Check sheet for the modelled part. Datum: model origin and axes. Units: mm. A direction names the side the tool comes from. Give positions to 0.01 mm unless a question says otherwise; leave off trailing zeros. Order: outer loops, then holes, each group sorted by start corner. A loop starts at its lowest first (then second) coordinate and runs counter-clockwise, first axis right, second up.
from build123d import *
from build123d import SkipClean  # not in build123d's __all__

# Parameters (mm, degrees)
F0_R     = 14.2875
F1_DEPTH = 3.175
F3_DEPTH = 15.875


with BuildPart() as f1:
    # F0 (on Front) → F1 (new body)
    with BuildSketch(Plane.XZ):
        with BuildLine():
            Line((-78.184375, -32.278895576), (-12.7, -49.1868884968))
            ThreePointArc((-12.7, -49.1868884968), (50.8, 0), (-12.7, 49.1868884968))
            Line((-12.7, 49.1868884968), (-78.184375, 32.278895576))
            ThreePointArc((-78.184375, 32.278895576), (-103.1875, 0), (-78.184375, -32.278895576))
        make_face()
        with Locations((-69.85, 0)):
            Circle(F0_R, mode=Mode.SUBTRACT)
        with BuildLine():
            ThreePointArc((-14.2875, 0), (0, 14.2875), (14.2875, 0))
            ThreePointArc((14.2875, 0), (0, -14.2875), (-14.2875, 0))
        make_face(mode=Mode.SUBTRACT)
    extrude(amount=F1_DEPTH)

    # F2 (on face) → F3 (join)
    with BuildSketch(Plane(origin=(0, 0, 0), x_dir=(-1, 0, 0), z_dir=(0, 1, 0))):
        with BuildLine():
            ThreePointArc((78.184375, -32.278895576), (103.1875, 0), (78.184375, 32.278895576))
            Line((78.184375, 32.278895576), (12.7, 49.1868884968))
            ThreePointArc((12.7, 49.1868884968), (-50.8, 0), (12.7, -49.1868884968))
            Line((12.7, -49.1868884968), (78.184375, -32.278895576))
        make_face()
        with BuildLine():
            Line((11.90625, 46.1127079658), (77.390625, 29.204715045))
            ThreePointArc((77.390625, 29.204715045), (100.0125, 0), (77.390625, -29.204715045))
            Line((77.390625, -29.204715045), (11.90625, -46.1127079658))
            ThreePointArc((11.90625, -46.1127079658), (-47.625, 0), (11.90625, 46.1127079658))
        make_face(mode=Mode.SUBTRACT)
    with SkipClean():  # cleaning this boolean's faces spoils the solid; the shape is the same uncleaned
        extrude(amount=F3_DEPTH)


solid = f1.part
1) Set-up check for faces 3 (the face through (-100.007, 7.826, 0.557)), 4 (the face through (-27, -3.175, 1)): record each of +Z, -Z, +X, -X, +Y, -Y from which the full face is reachable in a straight line by a thin tool's end or side.
Recorded:
face 3: +Y
face 4: +Z, -Z, +X, -X, -Y
2) Section check D-D, the plane x = 24.5. Record the cut outline in (y, z) (3 decimals).
Recorded:
outline: (-3.175, -44.502) - (15.875, -44.502) - (15.875, -40.84) - (0, -40.84) - (0, 40.84) - (15.875, 40.84) - (15.875, 44.502) - (-3.175, 44.502) - close
3) Section check B-B, the plane z = 0. Record the cut outline in (x, y) (1 decimal), then the cut area to 3 significant figures.
Recorded:
outline: (-103.2, -3.2) - (-84.1, -3.2) - (-84.1, 0) - (-100, 0) - (-100, 15.9) - (-103.2, 15.9) - close; (-55.6, -3.2) - (-14.3, -3.2) - (-14.3, 0) - (-55.6, 0) - close; (14.3, -3.2) - (50.8, -3.2) - (50.8, 15.9) - (47.6, 15.9) - (47.6, 0) - (14.3, 0) - close
area: 408 mm2
4) Material ranges on L1, parallel to Z at x = 0, y = 7.5 (3 decimals); L2, parallel to Z at x = 0, y = -1.1; L3, parallel to Y at x = 28.5, z = 27.5 (3 decimals), recorded low to high.
Recorded:
L1: z = -50.8 to -47.625, 47.625 to 50.8
L2: z = -50.8 to -14.29, 14.29 to 50.8
L3: y = -3.175 to 0
5) Section check A-A, the plane x = 0. Record the cut outline in (y, z) (1 decimal), then the cut area to 3 significant figures.
Recorded:
outline: (-3.2, -50.8) - (15.9, -50.8) - (15.9, -47.6) - (0, -47.6) - (0, -14.3) - (-3.2, -14.3) - close; (-3.2, 14.3) - (0, 14.3) - (0, 47.6) - (15.9, 47.6) - (15.9, 50.8) - (-3.2, 50.8) - close
area: 333 mm2
6) Depth check by flat-ended pin: pin 1 Ø2 at (y, z) = (1, 11) entering from -X; pin 2 Ø5 at (y, z) = (8, -7.5) entering from +X; pin 3 Ø4 at (x, y) = (-20, 13.5) entering from -Z; pin 4 Ø3 at (y, z) = (5, 1.5) entering from -X. Enter the tip coordinate at first touch or a pass-through.
Recorded:
pin 1: stops at x = -101.65
pin 2: stops at x = 50.55
pin 3: stops at z = -47.82
pin 4: stops at x = -103.19
7) Draft check along X on faces 1 (the face through (-20, 15.875, -45)), 2 (the face through (-45.11, 7.83, -37.54)). Enter one of: +X half, -X half, draft (parallel to the pull), parting line (faces both ways), or undercut.
Recorded:
face 1: draft
face 2: undercut
